from build123d import *

# Parameters (mm, degrees)
SKETCH1_R               = 19.05
SKETCH1_R_2             = 13.97
BOSS_EXTRUDE1_DEPTH     = 152.4
SKETCH2_R               = 13.97
BOSS_EXTRUDE2_DEPTH     = 6.35
SKETCH3_R               = 2.2479
CUT_EXTRUDE1_DEPTH      = 3.54
CUT_EXTRUDE1_DEPTH_BACK = 36.56
SKETCH5_W               = 10.16
SKETCH5_H               = 127
CUT_EXTRUDE5_DEPTH      = 20.0500001
CUT_EXTRUDE5_DEPTH_BACK = 20.0500001
SKETCH8_W               = 10.16
SKETCH8_H               = 127
CUT_EXTRUDE6_DEPTH      = 20.050000101
CUT_EXTRUDE6_DEPTH_BACK = 20.050000101
SKETCH7_R               = 6.35
CUT_EXTRUDE4_DEPTH      = 7.35
BOSS_EXTRUDE3_DEPTH     = 2.54


with BuildPart() as part:
    # Sketch1 → Boss-Extrude1 (new body)
    with BuildSketch(Plane(origin=(0, 0, 0), x_dir=(1, 0, 0), z_dir=(0, 1, 0))):
        Circle(SKETCH1_R)
        Circle(SKETCH1_R_2, mode=Mode.SUBTRACT)
    extrude(amount=BOSS_EXTRUDE1_DEPTH)

    # Sketch2 → Boss-Extrude2 (add)
    with BuildSketch(Plane.XZ):
        Circle(SKETCH2_R)
    extrude(amount=-BOSS_EXTRUDE2_DEPTH)

    # Sketch3 → Cut-Extrude1 (cut, two sides)
    with BuildSketch(Plane.XY.offset(16.51)) as cut_extrude1_sk:
        with Locations((0, 101.6)):
            Circle(SKETCH3_R)
    extrude(amount=CUT_EXTRUDE1_DEPTH, mode=Mode.SUBTRACT)
    extrude(cut_extrude1_sk.sketch, amount=-CUT_EXTRUDE1_DEPTH_BACK, mode=Mode.SUBTRACT)

    # Sketch5 → Cut-Extrude5 (cut, two sides)
    with BuildSketch(Plane(origin=(0, 0, 0), x_dir=(0, 0, -1), z_dir=(1, 0, 0))) as cut_extrude5_sk:
        with Locations((0, 76.2)):
            Rectangle(SKETCH5_W, SKETCH5_H)
    extrude(amount=CUT_EXTRUDE5_DEPTH, mode=Mode.SUBTRACT)
    extrude(cut_extrude5_sk.sketch, amount=-CUT_EXTRUDE5_DEPTH_BACK, mode=Mode.SUBTRACT)

    # Sketch8 → Cut-Extrude6 (cut, two sides)
    with BuildSketch(Plane.XY) as cut_extrude6_sk:
        with Locations((0, 76.2)):
            Rectangle(SKETCH8_W, SKETCH8_H)
    extrude(amount=CUT_EXTRUDE6_DEPTH, mode=Mode.SUBTRACT)
    extrude(cut_extrude6_sk.sketch, amount=-CUT_EXTRUDE6_DEPTH_BACK, mode=Mode.SUBTRACT)

    # Sketch7 → Cut-Extrude4 (cut, through all)
    with BuildSketch(Plane(origin=(0, 6.35, 0), x_dir=(1, 0, 0), z_dir=(0, 1, 0))):
        Circle(SKETCH7_R)
    extrude(amount=-CUT_EXTRUDE4_DEPTH, mode=Mode.SUBTRACT)

    # Sketch9 → Boss-Extrude3 (add)
    with BuildSketch(Plane(origin=(0, 45.72, 0), x_dir=(-1, 0, 0), z_dir=(0, -1, 0))):
        with BuildLine():
            Line((-11.787736325, -7.497344352), (-8.572899145, -5.452614074))
            ThreePointArc((-8.572899145, -5.452614074), (-6.7552586, -7.588944673), (-4.422740729, -9.14685544))
            Line((-4.422740729, -9.14685544), (-6.081268502, -12.57692623))
            ThreePointArc((-6.081268502, -12.57692623), (-9.288480575, -10.434798925), (-11.787736325, -7.497344352))
        make_face()
        with BuildLine():
            Line((11.787736325, 7.497344352), (8.572899145, 5.452614074))
            ThreePointArc((8.572899145, 5.452614074), (6.7552586, 7.588944673), (4.422740729, 9.14685544))
            Line((4.422740729, 9.14685544), (6.081268502, 12.57692623))
            ThreePointArc((6.081268502, 12.57692623), (9.288480575, 10.434798925), (11.787736325, 7.497344352))
        make_face()
    extrude(amount=-BOSS_EXTRUDE3_DEPTH)


solid = part.part
Geometry: final body of the model. Coordinates: model frame, mm. A direction names the side the tool comes from. Round coordinates to 2 decimals unless told otherwise and drop trailing zeros. Order: outer loops, then holes, each group sorted by start corner. A loop starts at its lowest first (then second) coordinate and runs counter-clockwise, first axis right, second up.
Q1. Pin query (flat end, axial travel): pin 1 (1.6 mm diameter, centred on x = 16, y = 91.5, fed in from +Z); pin 2 (10 mm diameter, centred on x = 1, y = 34, fed in from +Z); pin 3 (1.6 mm diameter, centred on x = -15.5, y = 102, fed in from -Z). Return the tip coordinate at first contact, or that it passes through.
Result sheet:
pin 1: stops at z = 11.48
pin 2: stops at z = 18.36
pin 3: stops at z = -12.12
Q2. Access query for faces 1 (the face through (-8, 45.72, -9)), 2 (the face through (-5, 0, 5)), 3 (the face through (16, 139.7, 0)), 4 (the face through (-8, 48.26, -9)), 5 (the face through (0, 12.7, -16)). Directions: +Z, -Z, +X, -X, +Y, -Y. A direction counts if a zero-diameter tool reaches every point of the face in a straight line with its end or side. Return the directions, or none.
Result sheet:
face 1: none
face 2: +Z, -Z, +X, -X, -Y
face 3: +X, -X
face 4: +Y
face 5: +Z, -Z
Q3. Section B-B, the plane x = 0. Output: boundary loops of the cut face in (y, z).
Result sheet:
outline: (0, -19.05) - (12.7, -19.05) - (12.7, -13.97) - (6.35, -13.97) - (6.35, -6.35) - (0, -6.35) - close; (0, 6.35) - (6.35, 6.35) - (6.35, 13.97) - (12.7, 13.97) - (12.7, 19.05) - (0, 19.05) - close; (139.7, -19.05) - (152.4, -19.05) - (152.4, -13.97) - (139.7, -13.97) - close; (139.7, 13.97) - (152.4, 13.97) - (152.4, 19.05) - (139.7, 19.05) - close
Q4. Section A-A, the plane y = 88. Output: boundary loops of the cut face in (x, z).
Result sheet:
outline: (-18.36, -5.08) arc R19.05 ccw to (-5.08, -18.36) - (-5.08, -13.01) arc R13.97 cw to (-13.01, -5.08) - close; (-18.36, 5.08) - (-13.01, 5.08) arc R13.97 cw to (-5.08, 13.01) - (-5.08, 18.36) arc R19.05 ccw to start; (5.08, -18.36) arc R19.05 ccw to (18.36, -5.08) - (13.01, -5.08) arc R13.97 cw to (5.08, -13.01) - close; (5.08, 13.01) arc R13.97 cw to (13.01, 5.08) - (18.36, 5.08) arc R19.05 ccw to (5.08, 18.36) - close
Q5. Material intervals for probe 1 along Z at (x, y) = (0, 4.5); probe 2 along Y at (x, z) = (2, 14), sorted ascending.
Result sheet:
probe 1: z = -19.05 to -6.35, 6.35 to 19.05
probe 2: y = 0 to 12.7, 139.7 to 152.4
Q6. Mould query, pull axis X, two halves, no side actions, for faces 6 (the face through (18.17, 75.13, -5.72)), 7 (the face through (16, 75, -5.08)), 8 (the face through (-6.785, 46.972, -7.563)). Classes: released by +X, released by -X, zero draft, split by the parting line, or undercut.
Result sheet:
face 6: split by the parting line
face 7: zero draft
face 8: undercut
Q7. Section C-C, the plane z = 3. Output: boundary loops of the cut face in (x, y).
Result sheet:
outline: (-18.81, 0) - (-5.6, 0) - (-5.6, 6.35) - (-13.64, 6.35) - (-13.64, 12.7) - (-18.81, 12.7) - close; (-18.81, 139.7) - (-13.64, 139.7) - (-13.64, 152.4) - (-18.81, 152.4) - close; (5.6, 0) - (18.81, 0) - (18.81, 12.7) - (13.64, 12.7) - (13.64, 6.35) - (5.6, 6.35) - close; (13.64, 139.7) - (18.81, 139.7) - (18.81, 152.4) - (13.64, 152.4) - close
